from build123d import *

# Parameters (mm, degrees)
SKETCH_1_R      = 10
SKETCH_1_R_2    = 3.5
EXTRUDE_1_DEPTH = 6.7
SKETCH_1_4_R    = 20
SKETCH_1_4_R_2  = 17
EXTRUDE_2_DEPTH = 12.64
SKETCH_1_5_R    = 17
SKETCH_1_5_R_2  = 10
EXTRUDE_3_DEPTH = 10.64
SKETCH_1_6_R    = 10
SKETCH_1_6_R_2  = 8
EXTRUDE_4_DEPTH = 17.64
FILLET_1_R      = 2


with BuildPart() as part:
    # 스케치1 → 보스-돌출1 (new body)
    with BuildSketch(Plane.XY):
        with BuildLine():
            Line((19.052558883, 11), (34.052558883, 6.5))
            Line((34.052558883, 6.5), (34.052558883, -6.5))
            Line((34.052558883, -6.5), (19.052558883, -11))
            ThreePointArc((19.052558883, -11), (0, -22), (-19.052558883, -11))
            Line((-19.052558883, -11), (-34.052558883, -6.5))
            Line((-34.052558883, -6.5), (-34.052558883, 6.5))
            Line((-34.052558883, 6.5), (-19.052558883, 11))
            ThreePointArc((-19.052558883, 11), (0, 22), (19.052558883, 11))
        make_face()
        Circle(SKETCH_1_R, mode=Mode.SUBTRACT)
        with Locations((26, 0)):
            Circle(SKETCH_1_R_2, mode=Mode.SUBTRACT)
        with Locations((-26, 0)):
            Circle(SKETCH_1_R_2, mode=Mode.SUBTRACT)
    extrude(amount=EXTRUDE_1_DEPTH)

    # 스케치1<4> → 보스-돌출2 (add)
    with BuildSketch(Plane.XY):
        with Locations(Location((0, 0, 0), (0, 0, 180))):
            Circle(SKETCH_1_4_R)
        with Locations(Location((0, 0, 0), (0, 0, 180))):
            Circle(SKETCH_1_4_R_2, mode=Mode.SUBTRACT)
    extrude(amount=EXTRUDE_2_DEPTH)

    # 스케치1<5> → 보스-돌출3 (add)
    with BuildSketch(Plane.XY):
        with Locations(Location((0, 0, 0), (0, 0, 180))):
            Circle(SKETCH_1_5_R)
        Circle(SKETCH_1_5_R_2, mode=Mode.SUBTRACT)
    extrude(amount=EXTRUDE_3_DEPTH)

    # 스케치1<6> → 보스-돌출4 (add)
    with BuildSketch(Plane.XY):
        Circle(SKETCH_1_6_R)
        Circle(SKETCH_1_6_R_2, mode=Mode.SUBTRACT)
    extrude(amount=EXTRUDE_4_DEPTH)

    # 필렛1
    fillet_1_edges = [part.edges().sort_by_distance(p)[0] for p in [
        (-34.052558883, -6.5, 3.35),
        (-34.052558883, 6.5, 3.35),
        (34.052558883, 6.5, 3.35),
        (34.052558883, -6.5, 3.35),
    ]]
    fillet(fillet_1_edges, radius=FILLET_1_R)


solid = part.part
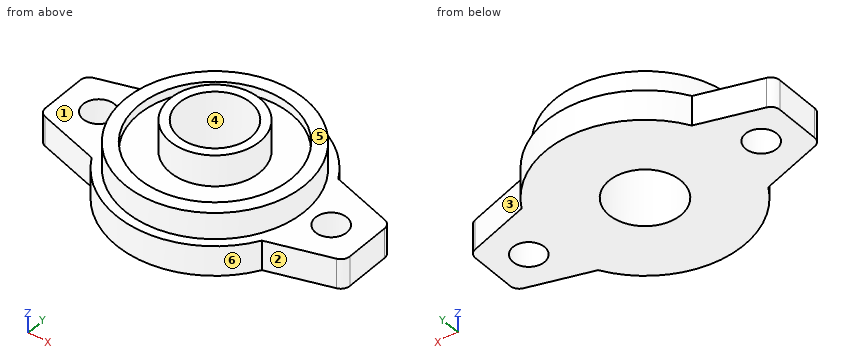
Could you check a few things on this model? Use its own coordinates, in mm. Face numbers are marked on the shaded views. A direction names the side the tool comes from. Round coordinates to 2 decimals unless told otherwise and drop trailing zeros. Loops run counter-clockwise (first coordinate to the right, second up) from the corner with the lowest first, then second, coordinate; pieces in that order, holes last. Notation, with made-up numbers: (-9, 29.5) - (29, 29.5) arc R21 ccw to (29, 58.5) - close; hole circle Ø8 at (55, 55). An arc over 180 degrees is marked (long way). Write item = value, one per line.
1) On a 3-axis mill with a long thin cutter (end or side, diameter ignored), from which of +Z, -Z, +X, -X, +Y, -Y can I reach the whole of each face in a straight line? I mean the marked faces 5 and 6. Say none if no direction works.
Computed:
face_5 = +Z
face_6 = +Z, -Z, -Y
2) Imagine slicing it at D-D (y = 6). Please give me the cut outline in (x, z).
Computed:
outline = (-33.79, 0) - (-5.29, 0) - (-5.29, 17.64) - (-8, 17.64) - (-8, 10.64) - (-15.91, 10.64) - (-15.91, 12.64) - (-19.08, 12.64) - (-19.08, 6.7) - (-33.79, 6.7) - close; (5.29, 0) - (33.79, 0) - (33.79, 6.7) - (19.08, 6.7) - (19.08, 12.64) - (15.91, 12.64) - (15.91, 10.64) - (8, 10.64) - (8, 17.64) - (5.29, 17.64) - close
3) I need wall thicknesses on line 1 along Y through (x, z) = (0, 11.2); line 2 along X through (y, z) = (-3, 12.5); line 3 along Y through (x, z) = (-3.5, 12.5). Which ranges of each line are inside material? Lowest first, please. Write a range as from..to.
Computed:
line_1 = -20..-17, -10..-8, 8..10, 17..20
line_2 = -19.77..-16.73, -9.54..-7.42, 7.42..9.54, 16.73..19.77
line_3 = -19.69..-16.64, -9.37..-7.19, 7.19..9.37, 16.64..19.69
4) Imagine slicing it at B-B (y = 0). Please give me the cut outline in (x, z), and give its area (3 significant figures).
Computed:
outline = (-34.05, 0) - (-29.5, 0) - (-29.5, 6.7) - (-34.05, 6.7) - close; (-22.5, 0) - (-8, 0) - (-8, 17.64) - (-10, 17.64) - (-10, 10.64) - (-17, 10.64) - (-17, 12.64) - (-20, 12.64) - (-20, 6.7) - (-22.5, 6.7) - close; (8, 0) - (22.5, 0) - (22.5, 6.7) - (20, 6.7) - (20, 12.64) - (17, 12.64) - (17, 10.64) - (10, 10.64) - (10, 17.64) - (8, 17.64) - close; (29.5, 0) - (34.05, 0) - (34.05, 6.7) - (29.5, 6.7) - close
area = 390 mm2
5) I'm going to push flat-ended pins straight in: P1, Ø1, axis at x = 13, y = 1, coming from the +Z side; P2, Ø10, axis at x = 26.5, y = 0, coming from the +Z side; P3, Ø4, axis at y = 6, z = 13, coming from the +X side. Where does each tip first touch, or does it pass through?
Computed:
P1 = 10.64
P2 = 6.7
P3 = 19.59
6) Imagine slicing it at A-A (x = 0). Please give me the cut outline in (y, z), and give its area (3 significant figures).
Computed:
outline = (-22, 0) - (-8, 0) - (-8, 17.64) - (-10, 17.64) - (-10, 10.64) - (-17, 10.64) - (-17, 12.64) - (-20, 12.64) - (-20, 6.7) - (-22, 6.7) - close; (8, 0) - (22, 0) - (22, 6.7) - (20, 6.7) - (20, 12.64) - (17, 12.64) - (17, 10.64) - (10, 10.64) - (10, 17.64) - (8, 17.64) - close
area = 322 mm2
7) Imagine slicing it at C-C (z = 3.25). Please give me the cut outline in (x, y).
Computed:
outline = (-34.05, -5.01) arc R2 ccw to (-32.63, -6.93) - (-19.05, -11) arc R22 ccw to (19.05, -11) - (32.63, -6.93) arc R2 ccw to (34.05, -5.01) - (34.05, 5.01) arc R2 ccw to (32.63, 6.93) - (19.05, 11) arc R22 ccw to (-19.05, 11) - (-32.63, 6.93) arc R2 ccw to (-34.05, 5.01) - close; hole circle Ø7 at (-26, 0); hole circle Ø16 at (0, 0); hole circle Ø7 at (26, 0)
8) If we mould it in two halves opening along Y, with no side actions, what happens to the marked faces 1, 2, 3 and 4? For each: pulls with the +Y half, pulls with the -Y half, needs draft (parallel to the pull), parting line crosses it, or undercut.
Computed:
face_1 = needs draft
face_2 = pulls with the -Y half
face_3 = pulls with the +Y half
face_4 = undercut
